from build123d import *

# Parameters (mm, degrees)
Y_KSEKLIK_EKSTR_ZYON1_DEPTH = 16
KES_EKSTR_ZYON1_DEPTH       = 97.432618963
KES_EKSTR_ZYON1_DEPTH_BACK  = 97.432618963
KES_EKSTR_ZYON2_DEPTH       = 97.432618963
KES_EKSTR_ZYON2_DEPTH_BACK  = 97.432618963
IZIM3_R                     = 8


with BuildPart() as part:
    # Çizim1 → Yükseklik-Ekstrüzyon1 (new, symmetric)
    with BuildSketch(Plane.XY):
        with BuildLine():
            Line((-33.5, 0), (33.5, 0))
            Line((33.5, 0), (33.5, -83.966738044))
            ThreePointArc((33.5, -83.966738044), (0, -89), (-33.5, -83.966738044))
            Line((-33.5, -83.966738044), (-33.5, 0))
        make_face()
    extrude(amount=Y_KSEKLIK_EKSTR_ZYON1_DEPTH, both=True)

    # Çizim2 → Kes-Ekstrüzyon1 (cut, two sides: drawn at the far end of the back side and taken through both)
    with BuildSketch(Plane(origin=(0, 0, 0), x_dir=(0, 0, -1), z_dir=(1, 0, 0)).offset(-KES_EKSTR_ZYON1_DEPTH_BACK)):
        with BuildLine():
            Line((-16, -16), (-16, 0))
            Line((-16, 0), (0, 0))
            ThreePointArc((0, 0), (-11.313708499, -4.686291501), (-16, -16))
        make_face()
    extrude(amount=KES_EKSTR_ZYON1_DEPTH + KES_EKSTR_ZYON1_DEPTH_BACK, mode=Mode.SUBTRACT)

    # Çizim3 → Kes-Ekstrüzyon2 (cut, two sides: drawn at the far end of the back side and taken through both)
    with BuildSketch(Plane(origin=(0, 0, 0), x_dir=(0, 0, -1), z_dir=(1, 0, 0)).offset(-KES_EKSTR_ZYON2_DEPTH_BACK)):
        with Locations((0, -16)):
            Circle(IZIM3_R)
    extrude(amount=KES_EKSTR_ZYON2_DEPTH + KES_EKSTR_ZYON2_DEPTH_BACK, mode=Mode.SUBTRACT)

    # Çizim4 → Kes-Döndür1 (revolve, cut)
    with BuildSketch(Plane(origin=(0, 0, 0), x_dir=(0, 0, -1), z_dir=(1, 0, 0)), mode=Mode.PRIVATE) as kes_d_nd_r1_sk:
        Polygon((-16, -34.5), (-3, -34.5), (-3, -39.5), (16, -39.5), (16, -56), (-16, -56), align=None)
    revolve(kes_d_nd_r1_sk.sketch.rotate(Axis((0, -56, 16), (0, 0, -1)), 90), axis=Axis((0, -56, 16), (0, 0, -1)), mode=Mode.SUBTRACT)


solid = part.part
Work out the finished part from the listing and answer in its coordinate system (mm). Coordinates: 2 decimals unless noted, no trailing zeros. Loops run counter-clockwise (first coordinate to the right, second up) from the corner with the lowest first, then second, coordinate; pieces in that order, holes last. Notation, with made-up numbers: (8.25, 53) -> (63.25, 53) arc R17 ccw to (63.25, 72) -> close; hole circle Ø10 at (-24.5, -6.5). An arc over 180 degrees is marked (long way). Write each question's results on one line, items separated by ' | '. Start each with the question number.
1) Find section C-C on y = -56. Determine the outline of the cut face in (x, z), then the cut area to 3 significant figures.
2) A flat-ended cylindrical pin translates along its axis: P1, Ø21.5, axis at x = 10, y = -55, coming from the +Z side. Find the tip coordinate at first contact, or state that the pin passes through.
3) Find section A-A on x = 0. Determine the outline of the cut face in (y, z).
4) The mould has two halves that part along X. Classify faces 1 (the cylindrical face through (-0.469, -4.563, 11.189)), 2 (the flat face through (-5, -40, 3)), 3 (the flat face through (33.5, -41, 0)), 4 (the cylindrical face through (-4.66, -35.01, 9.41)): pulls with the +X half, pulls with the -X half, needs draft (parallel to the pull), parting line crosses it, or undercut.
5) Find section D-D on x = -11. Determine the outline of the cut face in (y, z).
6) Consider line 1 along X through (y, z) = (-56, 9.5); line 2 along Y through (x, z) = (-7, -6.5); line 3 along Z through (x, y) = (14, -16). Determine where each line is inside the solid, lowest interval first.
7) Find section B-B on z = -4.5. Determine the outline of the cut face in (x, y), then the cut area to 3 significant figures.
Response values:
1) outline: (-33.5, -16) -> (-16.5, -16) -> (-16.5, 3) -> (-21.5, 3) -> (-21.5, 16) -> (-33.5, 16) -> close; (16.5, -16) -> (33.5, -16) -> (33.5, 16) -> (21.5, 16) -> (21.5, 3) -> (16.5, 3) -> close | area: 958 mm^2
2) P1: stops at z = 3
3) outline: (-89, -16) -> (-72.5, -16) -> (-72.5, 3) -> (-77.5, 3) -> (-77.5, 16) -> (-89, 16) -> close; (-39.5, -16) -> (0, -16) -> (0, 0) arc R16 ccw to (-16, 16) -> (-34.5, 16) -> (-34.5, 3) -> (-39.5, 3) -> close; hole circle Ø16 at (-16, 0)
4) face 1: needs draft | face 2: undercut | face 3: pulls with the +X half | face 4: undercut
5) outline: (-88.47, -16) -> (-68.3, -16) -> (-68.3, 3) -> (-74.47, 3) -> (-74.47, 16) -> (-88.47, 16) -> close; (-43.7, -16) -> (0, -16) -> (0, 0) arc R16 ccw to (-16, 16) -> (-37.53, 16) -> (-37.53, 3) -> (-43.7, 3) -> close; hole circle Ø16 at (-16, 0)
6) line 1: x = -33.5 to -21.5, 21.5 to 33.5 | line 2: y = -88.78 to -70.94, -41.06 to -20.66, -11.34 to 0 | line 3: z = -16 to -8, 8 to 16
7) outline: (-33.5, -83.97) arc R114 ccw to (33.5, -83.97) -> (33.5, -22.61) -> (-33.5, -22.61) -> close; (-33.5, -9.39) -> (33.5, -9.39) -> (33.5, 0) -> (-33.5, 0) -> close; hole circle Ø33 at (0, -56) | area: 4,110 mm^2
